from build123d import *

# Parameters (mm, degrees)
F0_R     = 15
F0_R_2   = 2
F1_DEPTH = 1.5
F2_R     = 3.85
F2_R_2   = 2
F3_DEPTH = 11.5
F4_DEPTH = 25


with BuildPart() as f1:
    # F0 (on Top) → F1 (new body)
    with BuildSketch(Plane.XY):
        Circle(F0_R)
        Circle(F0_R_2, mode=Mode.SUBTRACT)
    extrude(amount=F1_DEPTH)

    # F2 (on face) → F3 (join)
    with BuildSketch(Plane.XY.offset(1.5)):
        Circle(F2_R)
        Circle(F2_R_2, mode=Mode.SUBTRACT)
    extrude(amount=F3_DEPTH)

    # F4 (cut): a face of the model
    f4_faces = [f1.faces().sort_by_distance(p)[0] for p in [
        (-3.7411055557, 0, 13),
    ]]
    extrude(f4_faces, amount=-F4_DEPTH, mode=Mode.SUBTRACT)


solid = f1.part
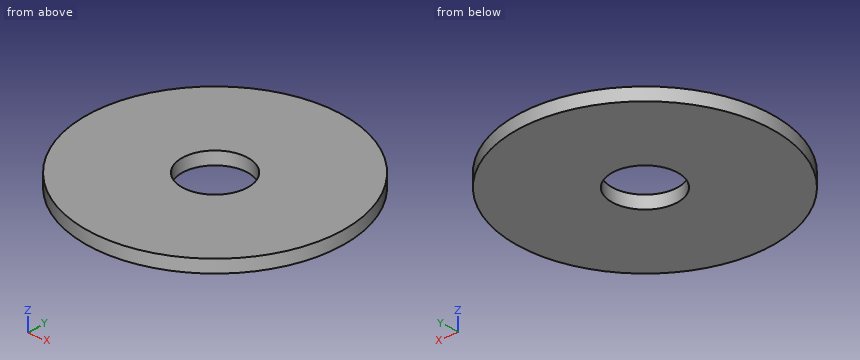
Build history of the part. All positions in model axes, mm. Give positions to 0.01 mm unless a question says otherwise; leave off trailing zeros. Loops run counter-clockwise (first coordinate to the right, second up) from the corner with the lowest first, then second, coordinate; pieces in that order, holes last. Notation, with made-up numbers: (27.25, 88) - (35.25, 88) arc R33 ccw to (35.25, 119) - close; hole circle Ø4 at (-33, 45.25). An arc over 180 degrees is marked (long way). Write item = value, one per line. Start each with the question number.
1) Band-saw the part on C-C on z = 0.3. Give the cut face in (x, y), plus the area to 3 significant figures.
2) Probe probe 1 along Y at (x, z) = (0, 0.8); probe 2 along Y at (x, z) = (3.5, 0.5); probe 3 along X at (y, z) = (-2.75, 1.15). List the from-to ranges inside material, lowest first. Write a range as from..to.
3) Band-saw the part on A-A on y = 0. Give the cut face in (x, z).
4) Band-saw the part on D-D on x = 11. Give the cut face in (y, z), plus the area to 3 significant figures.
5) Drop flat-ended pins along their axis: pin 1 Ø6 at (x, y) = (0, 0) entering from -Z; pin 2 Ø2 at (x, y) = (-8, -8) entering from -Z. Give the stop position or say it passes through.
Final values:
q1.outline = circle Ø30 at (0, 0); hole circle Ø7.7 at (0, 0)
q1.area = 660 mm²
q2.probe_1 = -15..-3.85, 3.85..15
q2.probe_2 = -14.59..-1.6, 1.6..14.59
q2.probe_3 = -14.75..-2.69, 2.69..14.75
q3.outline = (-15, 0) - (-3.85, 0) - (-3.85, 1.5) - (-15, 1.5) - close; (3.85, 0) - (15, 0) - (15, 1.5) - (3.85, 1.5) - close
q4.outline = (-10.2, 0) - (10.2, 0) - (10.2, 1.5) - (-10.2, 1.5) - close
q4.area = 30.6 mm²
q5.pin_1 = through
q5.pin_2 = 0
